from build123d import *

# Parameters (mm, degrees)
SKETCH_1_R      = 11.5
SKETCH_1_R_2    = 1.5
SKETCH_1_R_3    = 4
EXTRUDE_1_DEPTH = 5


with BuildPart() as part:
    # 草图1 → 凸台-拉伸1 (new body)
    with BuildSketch(Plane(origin=(0, 0, 0), x_dir=(0, 0, -1), z_dir=(1, 0, 0))):
        Polygon((-75, 75), (-88.5, 75), (-88.5, 72), (-87.25, 72), (-87.25, 69), (-88.5, 69), (-88.5, 67), (-91.5, 67), (-91.5, 69), (-92.75, 69), (-92.75, 72), (-91.5, 72), (-91.5, 75), (-105, 75), (-105, 65), (-100, 65), (-100, 45), (-105, 45), (-105, 30), (-100, 30), (-100, 10), (-105, 10), (-105, 0), (-75, 0), (-75, -5), (-35, -5), (-35, 0), (0, 0), (0, 10), (-5, 10), (-5, 30), (0, 30), (0, 45), (-5, 45), (-5, 65), (0, 65), (0, 75), (-16, 75), (-16, 72), (-14.75, 72), (-14.75, 69), (-16, 69), (-16, 67), (-19, 67), (-19, 69), (-20.25, 69), (-20.25, 72), (-19, 72), (-19, 75), (-35, 75), (-35, 80), (-75, 80), align=None)
        with Locations((-52.5, 37.5)):
            Circle(SKETCH_1_R, mode=Mode.SUBTRACT)
        with Locations((-68, 53)):
            Circle(SKETCH_1_R_2, mode=Mode.SUBTRACT)
        with Locations((-37, 53)):
            Circle(SKETCH_1_R_2, mode=Mode.SUBTRACT)
        with Locations((-37, 22)):
            Circle(SKETCH_1_R_2, mode=Mode.SUBTRACT)
        with Locations((-68, 22)):
            Circle(SKETCH_1_R_2, mode=Mode.SUBTRACT)
        with Locations((-39.5, 67.5)):
            Circle(SKETCH_1_R_3, mode=Mode.SUBTRACT)
        with Locations((-39.5, 7.5)):
            Circle(SKETCH_1_R_3, mode=Mode.SUBTRACT)
    extrude(amount=EXTRUDE_1_DEPTH)


solid = part.part
Build history of the part. All positions in model axes, mm. A direction names the side the tool comes from. Give positions to 0.01 mm unless a question says otherwise; leave off trailing zeros. Loops run counter-clockwise (first coordinate to the right, second up) from the corner with the lowest first, then second, coordinate; pieces in that order, holes last. Notation, with made-up numbers: (84.25, -18) -> (109.25, -18) arc R37 ccw to (109.25, 21) -> close; hole circle Ø8 at (38, -29). An arc over 180 degrees is marked (long way). Answer in a Markdown table with one row per item.
Item 1: Mould opens along Y. For faces 6 (the flat face through (2, 30, 3)), 7 (the flat face through (2, 70, 105)), 8 (the flat face through (2, 75, 82)) say: pulls with the +Y half, pulls with the -Y half, needs draft (parallel to the pull), parting line crosses it, or undercut.
Findings below:
| item | result |
|---|---|
| face 6 | undercut |
| face 7 | needs draft |
| face 8 | pulls with the +Y half |
Item 2: Slice it at A-A on z = 52.5. Write the cut outline in (x, y).
Findings below:
| item | result |
|---|---|
| outline | (0, -5) -> (5, -5) -> (5, 26) -> (0, 26) -> close; (0, 49) -> (5, 49) -> (5, 80) -> (0, 80) -> close |
Item 3: Tool access for faces 1 (the flat face through (2, 65, 3)), 2 (the flat face through (2, 73, 91.5)), 3 (the flat face through (2, 75, 27)), 4 (the flat face through (2, 30, 103)), 5 (the flat face through (2, 71, 14.75)): list every direction of +Z, -Z, +X, -X, +Y, -Y with a clear straight run to the whole face (end or side of a thin tool).
Findings below:
| item | result |
|---|---|
| face 1 | -Z, +X, -X |
| face 2 | +X, -X, +Y |
| face 3 | -Z, +X, -X, +Y |
| face 4 | +Z, +X, -X |
| face 5 | +X, -X |
Item 4: Slice it at C-C on y = 22. Write the cut outline in (x, z), plus the area to 3 significant figures.
Findings below:
| item | result |
|---|---|
| outline | (0, 5) -> (5, 5) -> (5, 35.5) -> (0, 35.5) -> close; (0, 38.5) -> (5, 38.5) -> (5, 66.5) -> (0, 66.5) -> close; (0, 69.5) -> (5, 69.5) -> (5, 100) -> (0, 100) -> close |
| area | 445 mm² |
Item 5: Probe line 1 along Y through (x, z) = (1.75, 68); line 2 along Y through (x, z) = (1.15, 39.5); line 3 along Y through (x, z) = (2.75, 37). List the from-to ranges inside material, lowest first. Write a range as [from, to].
Findings below:
| item | result |
|---|---|
| line 1 | y = [-5, 20.5], [23.5, 51.5], [54.5, 80] |
| line 2 | y = [-5, 3.5], [11.5, 63.5], [71.5, 80] |
| line 3 | y = [-5, 4.38], [10.62, 20.5], [23.5, 51.5], [54.5, 64.38], [70.62, 80] |
Item 6: Slice it at D-D on z = 79.5. Write the cut outline in (x, y).
Findings below:
| item | result |
|---|---|
| outline | (0, 0) -> (5, 0) -> (5, 75) -> (0, 75) -> close |
Item 7: Flat gauge pins, fed straight in: P1, Ø1.5, axis at x = 1.5, y = 77, coming from the -Z side; P2, Ø1.8, axis at y = 53, z = 37, coming from the +X side; P3, Ø1.4, axis at x = 3.5, z = 92.5, coming from the +Y side; P4, Ø0.6, axis at x = 1.5, z = 15.5, coming from the -Y side. Where does each tip first touch, or does it go through?
Findings below:
| item | result |
|---|---|
| P1 | stops at z = 35 |
| P2 | passes through |
| P3 | stops at y = 75 |
| P4 | stops at y = 0 |
Item 8: Slice it at B-B on y = 7.5. Write the cut outline in (x, z), plus the area to 3 significant figures.
Findings below:
| item | result |
|---|---|
| outline | (0, 0) -> (5, 0) -> (5, 35.5) -> (0, 35.5) -> close; (0, 43.5) -> (5, 43.5) -> (5, 105) -> (0, 105) -> close |
| area | 485 mm² |
